Can you work these out from the model? Positions are in its coordinate system, mm. A direction names the side the tool comes from. Coordinates: 2 decimals unless noted, no trailing zeros. Order: outer loops, then holes, each group sorted by start corner. A loop starts at its lowest first (then second) coordinate and runs counter-clockwise, first axis right, second up. Notation, with made-up numbers: (34.5, 2.5) -> (92.5, 2.5) arc R10 cw to (92.5, 19.5) -> close; hole circle Ø8 at (8, 16). An arc over 180 degrees is marked (long way). Write item = value, one per line. Start each with the question number.
from build123d import *

# Parameters (mm, degrees)
SKETCH1_R               = 11
BOSS_EXTRUDE1_DEPTH     = 16.875
SKETCH2_R               = 10
BOSS_EXTRUDE2_DEPTH     = 14.0625
SKETCH3_R               = 10
BOSS_EXTRUDE3_DEPTH     = 14.0625
CUT_EXTRUDE4_DEPTH      = 15.0625
CUT_EXTRUDE4_DEPTH_BACK = 31.9375
SKETCH6_W               = 1
SKETCH6_H               = 0.5
F_3_8_24_TAPPED_HOLE1_D = 8.4328
SKETCH10_R              = 3.175
CUT_EXTRUDE5_DEPTH      = 1
CUT_EXTRUDE5_DEPTH_BACK = 46
CHAMFER1_SIZE           = 1


with BuildPart() as part:
    # Sketch1 → Boss-Extrude1 (new body)
    with BuildSketch(Plane.XY):
        Circle(SKETCH1_R)
    extrude(amount=BOSS_EXTRUDE1_DEPTH)

    # Sketch2 → Boss-Extrude2 (add)
    with BuildSketch(Plane(origin=(0, 0, 0), x_dir=(-1, 0, 0), z_dir=(0, 0, -1))):
        Circle(SKETCH2_R)
    extrude(amount=BOSS_EXTRUDE2_DEPTH)

    # Sketch3 → Boss-Extrude3 (add)
    with BuildSketch(Plane.XY.offset(16.875)):
        Circle(SKETCH3_R)
    extrude(amount=BOSS_EXTRUDE3_DEPTH)

    # Sketch5 → Cut-Extrude4 (cut, two sides)
    with BuildSketch(Plane(origin=(0, 0, 0), x_dir=(-1, 0, 0), z_dir=(0, 0, -1))) as cut_extrude4_sk:
        with BuildLine():
            Line((-10, -4.582575695), (-10, 4.582575695))
            ThreePointArc((-10, 4.582575695), (-11, 0), (-10, -4.582575695))
        make_face()
        with BuildLine():
            ThreePointArc((11, 0), (10.74709263, 2.34520788), (10, 4.582575695))
            Line((10, 4.582575695), (10, -4.582575695))
            ThreePointArc((10, -4.582575695), (10.74709263, -2.34520788), (11, 0))
        make_face()
    extrude(amount=CUT_EXTRUDE4_DEPTH, mode=Mode.SUBTRACT)
    extrude(cut_extrude4_sk.sketch, amount=-CUT_EXTRUDE4_DEPTH_BACK, mode=Mode.SUBTRACT)

    # Sketch6 → Cut-Revolve1 (revolve, cut)
    with BuildSketch(Plane(origin=(0, 0, 0), x_dir=(0, 0, -1), z_dir=(1, 0, 0))):
        with Locations((12.5625, 9.75)):
            Rectangle(SKETCH6_W, SKETCH6_H)
        with BuildLine():
            Line((-15.875, 11), (-13.875, 11))
            ThreePointArc((-13.875, 11), (-14.875, 10), (-15.875, 11))
        make_face()
        with Locations((-29.4375, 9.75)):
            Rectangle(SKETCH6_W, SKETCH6_H)
        with BuildLine():
            Line((-3, 11), (-1, 11))
            ThreePointArc((-1, 11), (-2, 10), (-3, 11))
        make_face()
    revolve(axis=Axis((0, 0, 30.9375), (0, 0, -1)), mode=Mode.SUBTRACT)

    # 3/8-24 Tapped Hole1 (through all)
    with Locations(Plane(origin=(10, 0, 0), x_dir=(0, 0, -1), z_dir=(1, 0, 0))):
        with Locations((-8.4375, 0)):
            Hole(F_3_8_24_TAPPED_HOLE1_D / 2)

    # Sketch10 → Cut-Extrude5 (cut, two sides)
    with BuildSketch(Plane(origin=(0, 0, -14.0625), x_dir=(-1, 0, 0), z_dir=(0, 0, -1))) as cut_extrude5_sk:
        Circle(SKETCH10_R)
    extrude(amount=CUT_EXTRUDE5_DEPTH, mode=Mode.SUBTRACT)
    extrude(cut_extrude5_sk.sketch, amount=-CUT_EXTRUDE5_DEPTH_BACK, mode=Mode.SUBTRACT)

    # Chamfer1
    chamfer1_edges = [part.edges().sort_by_distance(p)[0] for p in [
        (3.175, 0, -14.0625),
        (3.175, 0, 30.9375),
    ]]
    chamfer(chamfer1_edges, length=CHAMFER1_SIZE)


solid = part.part
(1) For faces 1 (the face through (-9.54, 3, -13.56)), 2 (the face through (-2, -10, 16.875)), 3 (the face through (-2, 10, 0)), 4 (the face through (0.2, 11, 0.5)), 5 (the face through (-2, -10, 0)), which set-ups out of +Z, -Z, +X, -X, +Y, -Y let a thin tool reach every point of the face, with its end or its side?
(2) Imagine slicing it at A-A (z = 7). Write out the boundary of the cut face in (x, y).
(3) For P1, Ø1.5, axis at y = -6.5, z = -3.5, coming from the -X side; P2, Ø2, axis at x = -7.5, y = -7, coming from the -Z side; P3, Ø8, axis at x = 5, z = -1.5, coming from the -Y side; P4, Ø5.5, axis at x = 0, y = 0, coming from the -Z side, each with a flat end and sliding along its axis, tell me the tip position at first contact or that it passes through.
(4) Imagine slicing it at B-B (z = 2.5). Write out the boundary of the cut face in (x, y) (3 decimals), plus the area to 3 significant figures.
(5) Thinking about a two-plate mould opening in X: for faces 6 (the face through (10, 0, 1)), 7 (the face through (3.17, 0.14, -3.83)), 8 (the face through (0, -11, 8)), 9 (the face through (-4, -9, 28.938)), which applies, +X half, -X half, draft (parallel to the pull), parting line (faces both ways), or undercut?
(6) If I drill on L1, parallel to X at y = 0.25, z = -5; L2, parallel to Y at x = 0, z = -5.25 (3 decimals); L3, parallel to Z at x = 3.75, y = 10 (3 decimals), over which ranges is the centre line in solid material (lowest first)? Write a range as from..to.
Result set:
q1.face_1 = -Z
q1.face_2 = +Z, -Y
q1.face_3 = -Z, +Y
q1.face_4 = +Z, -Z, +Y
q1.face_5 = -Z, -Y
q2.outline = (-10, -4.58) arc R11 ccw to (10, -4.58) -> (10, -3.96) -> (-10, -3.96) -> close; (-10, 3.96) -> (10, 3.96) -> (10, 4.58) arc R11 ccw to (-10, 4.58) -> close
q3.P1 = -8.18
q3.P2 = -14.06
q3.P3 = -10.92
q3.P4 = through
q4.outline = (-10, -1.642) arc R10.134 ccw to (10, -1.642) -> (10, 1.642) arc R10.134 ccw to (-10, 1.642) -> close; hole circle Ø6.35 at (0, 0)
q4.area = 290 mm2
q5.face_6 = +X half
q5.face_7 = undercut
q5.face_8 = parting line
q5.face_9 = draft
q6.L1 = -10..-3.17, 3.17..10
q6.L2 = -10..-3.175, 3.175..10
q6.L3 = 0..1.053, 2.947..13.928, 15.822..16.875
